Source: CAD feature listing. Evaluate the final solid. Frame: model axes, mm. A direction names the side the tool comes from. Give positions to 0.01 mm unless a question says otherwise; leave off trailing zeros. Order: outer loops, then holes, each group sorted by start corner. A loop starts at its lowest first (then second) coordinate and runs counter-clockwise, first axis right, second up.
Autodesk Inventor part; units mm, degrees
ref_plane "YZ Plane" through (0, 0, 0) normal (1, 0, 0) x (0, 1, 0)
ref_plane "XZ Plane" through (0, 0, 0) normal (0, 1, 0) x (-1, 0, 0)
ref_plane "XY Plane" through (0, 0, 0) normal (0, 0, 1) x (1, 0, 0)
sketch "Skizze1" plane through (0, 0, 0) normal (0, 0, 1) x (1, 0, 0)
  line L0 (0, 0) -> (6.75, 0)
  line L1 (6.75, 0) -> (6.75, 4.9)
  line L2 (6.75, 4.9) -> (3.75, 4.9)
  line L3 (3.75, 4.9) -> (3.75, 10.2)
  line L4 (3.75, 10.2) -> (18.25, 10.2)
  line L5 (18.25, 10.2) -> (18.25, 4.9)
  line L6 (18.25, 4.9) -> (15.25, 4.9)
  line L7 (15.25, 4.9) -> (15.25, 0)
  line L8 (15.25, 0) -> (22, 0)
  line L9 (22, 0) -> (22, 80.2)
  line L10 (0, 0) -> (0, 64.9782)
  line L11 (22, 80.2) -> (22, 98.8308) construction
  line L12 (22, 80.2) -> (20.0304, 79.8527)
  line L13 (20.0304, 79.8527) -> (18.8148, 86.7464)
  arc A0 (22, 86.9782) -> (18.8148, 86.7464) centre (22, 64.9782) ccw construction
  arc A1 (18.8148, 86.7464) -> (0, 64.9782) centre (22, 64.9782) ccw
  dimension "d0" = 14.5
  dimension "d1" = 5.3
  dimension "d2" = 4.9
  dimension "d3" = 22
  dimension "d4" = 8.5
  dimension "d5" = 2
  dimension "d6" = 7
  dimension "d21" = 70
  dimension "d22" = 80
extrude "Extrusion1" add sketch "Skizze1" along normal blind 22
sketch "Skizze2" plane through (22, 0, 0) normal (1, 0, 0) x (0, 0, -1)
  circle A0 centre (-11, 7.5) radius 2
  line L0 (0, 0) -> (-22, 0)
  line L1 (0, 0) -> (0, 80.2)
  point P0 (0, 65.2)
  dimension "d10" = 4
  dimension "d11" = 7.5
  dimension "d12" = 11
extrude "Extrusion2" cut sketch "Skizze2" against normal blind 22
chamfer "Fasen1" distance 1 angle 45 18 edges at (3.75, 7.55, 22) (11, 10.2, 22) (18.25, 7.55, 22) (16.75, 4.9, 22) (5.25, 4.9, 22) (6.75, 2.45, 22) (15.25, 2.45, 22) (18.25, 7.55, 0) (15.25, 2.45, 0) (16.75, 4.9, 0) (11, 10.2, 0) (3.75, 7.55, 0) (5.25, 4.9, 0) (6.75, 2.45, 0) (6.75, 4.9, 11) (15.25, 4.9, 11) (6.75, 0, 11) (15.25, 0, 11)
sketch "Skizze3" plane through (20.0304, 79.8527, 22) normal (-0.1736, 0.9848, 0) x (0.9848, 0.1736, 0)
  circle A0 centre (4, 11) radius 6 construction
  line L0 (0, 6.5147) -> (-4.4853, 11)
  line L1 (-4.4853, 11) -> (0, 15.4853)
  line L2 (0, 15.4853) -> (0, 6.5147)
  line L3 (2, 22) -> (2, 0)
  line L4 (0, 22) -> (0, 0)
  point P0 (-33.5924, 22)
  point P1 (0, 11)
  dimension "d23" = 12
  dimension "d24" = 45
  dimension "d26" = 4
extrude "Extrusion3" cut sketch "Skizze3" along normal blind 10
properties part number "Gripper_V2_10deg"
1) Draft query along Y for faces 1 (the flat face through (0, 32, 11)), 2 (the flat face through (5, 4.9, 11)), 3 (the flat face through (3, 0, 11)). Return one class per face: +Y half, -Y half, draft (parallel to the pull), parting line (faces both ways), or undercut.
Report:
face 1: draft
face 2: undercut
face 3: -Y half
2) Section query C-C, the plane x = 8. Return the cut outline in (y, z), and give its area (3 significant figures).
Report:
outline: (10.2, 1) - (11.2, 0) - (81.95, 0) - (81.95, 22) - (11.2, 22) - (10.2, 21) - close
area: 1,580 mm2
3) Pin query (flat end, axial travel): pin 1 (6 mm diameter, centred on x = 7, z = 6, fed in from +Y); pin 2 (1 mm diameter, centred on x = 17, z = 7, fed in from +Y); pin 3 (1.5 mm diameter, centred on x = 12, y = 74, fed in from -Z); pin 4 (1.6 mm diameter, centred on x = 4.5, z = 7.5, fed in from +Y). Return the tip coordinate at first contact, or that it passes through.
Report:
pin 1: stops at y = 83.42
pin 2: stops at y = 86.51
pin 3: stops at z = 0
pin 4: stops at y = 79.3
4) Reachability of faces 4 (the flat face through (18.28, 79.54, 10.94)), 5 (the flat face through (6.75, 2, 11)), 6 (the flat face through (19, 0, 11)), 7 (the flat face through (21.03, 80.03, 10.85)), 8 (the flat face through (17, 4.9, 11)) from +Z, -Z, +X, -X, +Y, -Y: full face, straight path, thin tool, end or side. Return the list, or none.
Report:
face 4: +Y
face 5: +Z, -Z, -Y
face 6: +Z, -Z, +X, -X, -Y
face 7: +Z, -Z, +Y
face 8: +Z, -Z
5) Section query D-D, the plane y = 75.5. Return the cut outline in (x, z), and give its area (3 significant figures).
Report:
outline: (2.68, 0) - (22, 0) - (22, 22) - (2.68, 22) - close
area: 425 mm2
6) Section query A-A, the plane y = 7.5. Return the cut outline in (x, z), and give its area (3 significant figures).
Report:
outline: (0, 0) - (2.75, 0) - (3.75, 1) - (3.75, 9) - (0, 9) - close; (0, 13) - (3.75, 13) - (3.75, 21) - (2.75, 22) - (0, 22) - close; (18.25, 1) - (19.25, 0) - (22, 0) - (22, 9) - (18.25, 9) - close; (18.25, 13) - (22, 13) - (22, 22) - (19.25, 22) - (18.25, 21) - close
area: 133 mm2
7) Section query B-B, the plane z = 20.25. Return the cut outline in (x, y).
Report:
outline: (0, 0) - (5.75, 0) - (6.75, 1) - (6.75, 3.9) - (5.75, 4.9) - (3.75, 4.9) - (3.75, 10.2) - (18.25, 10.2) - (18.25, 4.9) - (16.25, 4.9) - (15.25, 3.9) - (15.25, 1) - (16.25, 0) - (22, 0) - (22, 80.2) - (20.03, 79.85) - (18.81, 86.75) arc R22 ccw to (0, 64.98) - close
8) Material intervals for L1, parallel to Y at x = 6.5, z = 1; L2, parallel to Y at x = 20.25, z = 11.75; L3, parallel to Y at x = 8.75, z = 13.75, sorted ascending.
Report:
L1: y = 0.75 to 4.15, 10.2 to 80.59
L2: y = 0 to 5.65, 9.35 to 79.89
L3: y = 10.2 to 82.54
